from build123d import *

# Parameters (mm, degrees)
F2_W     = 63.1503015757
F2_H     = 7.9845217988
F5_R     = 32.2206110424
F6_DEPTH = 279.4


with BuildPart() as f3:
    # F0 (on Front) → F3 section 0
    with BuildSketch(Plane.XZ):
        with BuildLine():
            ThreePointArc((23.0088164468, 21.8782281211), (0.6907278555, 31.7424856467), (-22.0353312907, 22.8584049074))
            ThreePointArc((-22.0353312907, 22.8584049074), (-31.6817312095, 2.0809631345), (-24.8359487489, -19.7797408917))
            ThreePointArc((-24.8359487489, -19.7797408917), (1.096665301, -31.7310545872), (26.1422818553, -18.0178688917))
            ThreePointArc((26.1422818553, -18.0178688917), (31.6525236796, 2.4860097971), (23.0088164468, 21.8782281211))
        make_face()
    # F2 (on offset) → F3 section 1
    with BuildSketch(Plane.XZ.offset(88.9)):
        Rectangle(F2_W, F2_H)
    loft()

    # F5 (on offset) → F6 (join)
    with BuildSketch(Plane.XZ):
        Circle(F5_R)
    extrude(amount=-F6_DEPTH)

    # F7 (on Right) → F8 (revolve)
    with BuildSketch(Plane.YZ):
        with BuildLine():
            add(Edge.make_bspline(
                [(278.835952282, 32.7780023217), (277.8359174772, 36.6024541602), (275.2821107075, 46.3690252322), (300.2033188051, 27.9764485938), (333.2199939586, 46.1555304856), (369.4104964708, 56.2417917829), (421.3321098132, 60.7266040333), (442.145049702, 33.9653899591), (443.34846302, 10.4804242711), (443.2389499023, 2.9934523278), (443.1951642036, 0)],
                knots=[0, 0, 0, 0, 0.0724523247, 0.1850227977, 0.3345498986, 0.4926059997, 0.6664305507, 0.8025875127, 0.9210702439, 1, 1, 1, 1], degree=3))
            Line((278.835952282, 32.7780023217), (278.835952282, 0))
            Line((278.835952282, 0), (443.1951642036, 0))
        make_face()
    revolve(axis=Axis((0, 361.0155582428, 0), (0, 1, 0)))


solid = f3.part
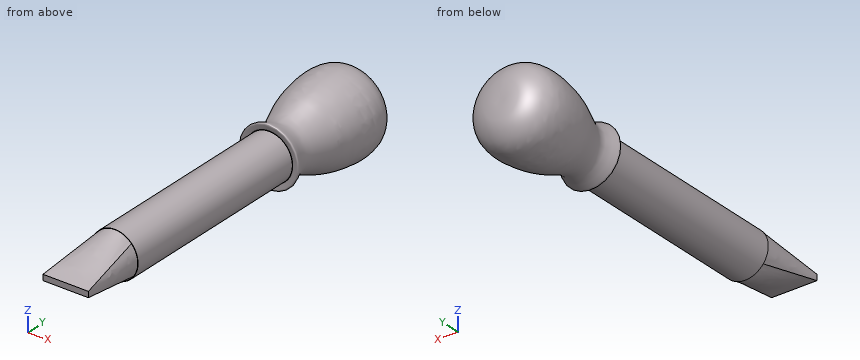
The listing builds one solid part. Answer for the finished solid, in the listing's coordinates (mm). Round coordinates to 2 decimals unless told otherwise and drop trailing zeros. Order: outer loops, then holes, each group sorted by start corner. A loop starts at its lowest first (then second) coordinate and runs counter-clockwise, first axis right, second up. Notation, with made-up numbers: (-29.75, 24.25) - (15.25, 24.25) arc R20 cw to (15.25, 40.25) - close; hole circle Ø1 at (51, 78.25). An arc over 180 degrees is marked (long way). Write item = value, one per line. Start each with the question number.
1) Section A-A, the plane y = 130 is taken. Write down the section's boundary in (x, z), plus the area to 3 significant figures.
2) Straight lines are drawn through the part: L1, parallel to Y at x = -37, z = 16.5; L2, parallel to X at y = 274.5, z = 2.5; L3, parallel to Y at x = -40, z = 6.5. For each, find the intervals that lie inside material, in ascending order.
3) Given pin 1 (12 mm diameter, centred on x = 41.5, z = -14.5, fed in from +Y); pin 2 (5 mm diameter, centred on y = 217.5, z = 9, fed in from -X); pin 3 (1 mm diameter, centred on y = 3.5, z = -29, fed in from -X), each flat-ended and moving along its own axis, determine where each tip first touches the part or whether it passes through.
Results list:
q1.outline = circle Ø64.44 at (0, 0)
q1.area = 3,260 mm^2
q2.L1 = 277.76 to 282.14, 323.94 to 435.63
q2.L2 = -32.12 to 32.12
q2.L3 = 277.77 to 282.11, 323.97 to 435.62
q3.pin_1 = 437.15
q3.pin_2 = -31.56
q3.pin_3 = -15.03
